Input: dimensioned drawing with shaded views. Units: mm. Origin: part minimum x, y, z. Give positions to 0.01 mm unless a question says otherwise; leave off trailing zeros. Order: outer loops, then holes, each group sorted by start corner. A loop starts at its lowest first (then second) coordinate and runs counter-clockwise, first axis right, second up.
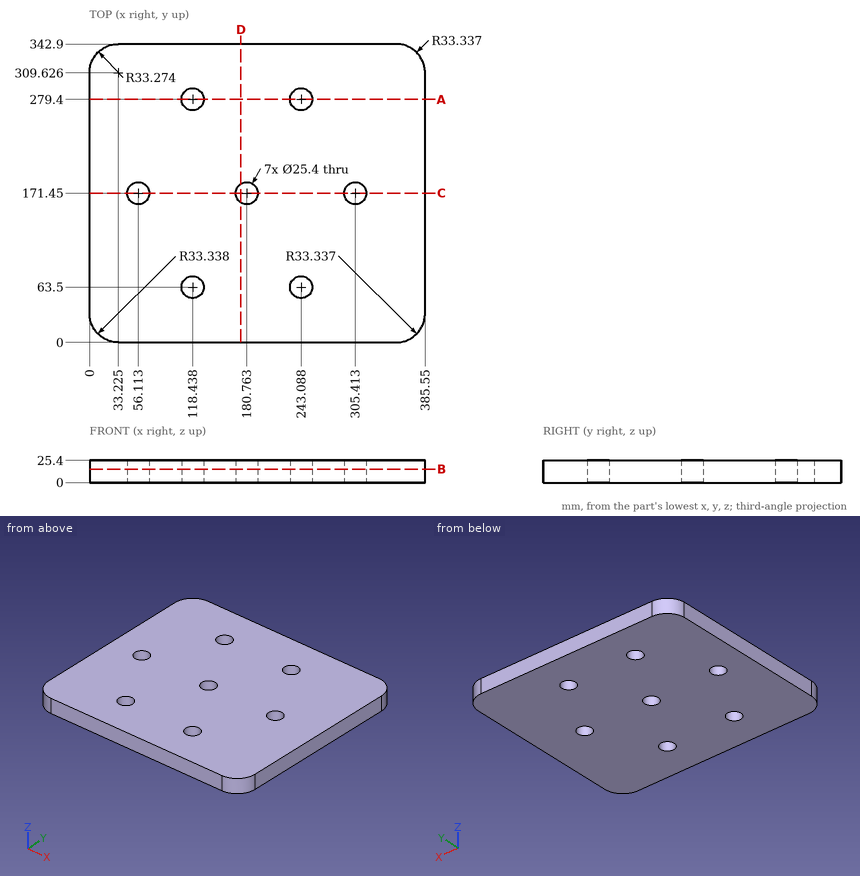
1) Section query A-A, the plane y = 279.4. Return the cut outline in (x, z).
Report:
outline: (0, 0) - (105.74, 0) - (105.74, 25.4) - (0, 25.4) - close; (131.14, 0) - (230.39, 0) - (230.39, 25.4) - (131.14, 25.4) - close; (255.79, 0) - (385.55, 0) - (385.55, 25.4) - (255.79, 25.4) - close
2) Section query D-D, the plane x = 174. Return the cut outline in (y, z).
Report:
outline: (0, 0) - (160.7, 0) - (160.7, 25.4) - (0, 25.4) - close; (182.2, 0) - (342.9, 0) - (342.9, 25.4) - (182.2, 25.4) - close
3) Section query B-B, the plane z = 15.5. Count the separate pieces of the cut face and the enclosed holes in it, and give its area (3 significant figures).
Report:
separate pieces: 1
enclosed holes: 7
area: 128,000 mm2
4) Material intervals for L1, parallel to Y at x = 250, z = 14.25 (1 decimal); L2, parallel to Y at x = 109.5, z = 8.25 (1 decimal); L3, parallel to Y at x = 60, z = 9.75, sorted ascending.
Report:
L1: y = 0 to 52.8, 74.2 to 268.7, 290.1 to 342.9
L2: y = 0 to 54.5, 72.5 to 270.4, 288.4 to 342.9
L3: y = 0 to 159.36, 183.54 to 342.9
5) Section query C-C, the plane y = 171.45. Return the cut outline in (x, z).
Report:
outline: (0, 0) - (43.41, 0) - (43.41, 25.4) - (0, 25.4) - close; (68.81, 0) - (168.06, 0) - (168.06, 25.4) - (68.81, 25.4) - close; (193.46, 0) - (292.71, 0) - (292.71, 25.4) - (193.46, 25.4) - close; (318.11, 0) - (385.55, 0) - (385.55, 25.4) - (318.11, 25.4) - close
